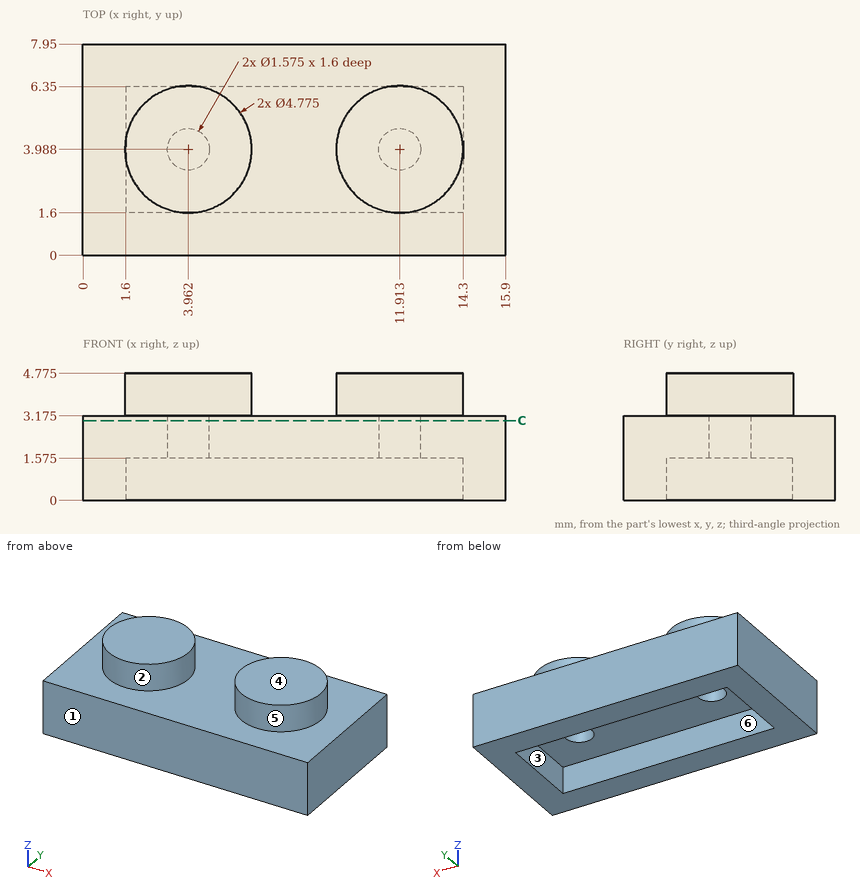
Drawing for the job (mm, zero at the part's lowest x, y, z). A direction names the side the tool comes from. Round coordinates to 2 decimals unless told otherwise and drop trailing zeros. Use one line per item in the form item = value. Start each with the question number.
Item 1: Tool access for the marked faces 4, 5 and 6: list every direction of +Z, -Z, +X, -X, +Y, -Y with a clear straight run to the whole face (end or side of a thin tool).
Item 2: Drop flat-ended pins along their axis: pin 1 Ø1 at (y, z) = (1.5, 4) entering from +X (1 decimal); pin 2 Ø1.4 at (x, y) = (3.96, 3.99) entering from -Z (3 decimals); pin 3 Ø1.3 at (x, y) = (12, 3.5) entering from -Z (1 decimal). Give the stop position or say it passes through.
Item 3: Two-plate mould, pull along Y, no slides. Class the marked faces 1, 2 and 3: released by +Y, released by -Y, zero draft, split by the parting line, or undercut.
Item 4: Band-saw the part on C-C (z = 3). Give the number of separate pieces and of enclosed holes in the cut face.
Item 5: Drill centre lines: line 1 along Y through (x, z) = (9.25, 0.25); line 2 along X through (y, z) = (4.25, 2.8) (1 decimal); line 3 along Z through (x, y) = (12.25, 7.75) (1 decimal). Where is each one in solid material? Low to high.
Data:
q1.face_4 = +Z, +X, -X, +Y, -Y
q1.face_5 = +Z
q1.face_6 = -Z
q2.pin_1 = 13.2
q2.pin_2 = 3.175
q2.pin_3 = 1.6
q3.face_1 = released by -Y
q3.face_2 = split by the parting line
q3.face_3 = undercut
q4.separate_pieces = 1
q4.enclosed_holes = 2
q5.line_1 = 0 to 1.6, 6.35 to 7.95
q5.line_2 = 0 to 3.2, 4.7 to 11.2, 12.7 to 15.9
q5.line_3 = 0 to 3.2
